from build123d import *
from build123d.topology import SkipClean

# Parameters (mm, degrees)
SKETCH1_R           = 7
BOSS_EXTRUDE1_DEPTH = 20
SKETCH2_R           = 13.25
CUT_EXTRUDE1_DEPTH  = 14
SKETCH3_R           = 4
CUT_EXTRUDE2_DEPTH  = 76.40989747
SKETCH4_W           = 110
SKETCH4_H           = 5
BOSS_EXTRUDE2_DEPTH = 10
SKETCH5_W           = 110
SKETCH5_H           = 5
BOSS_EXTRUDE3_DEPTH = 10
FILLET1_START       = -40
FILLET1_DEPTH       = 80
FILLET1_START_2     = -10.0000001
FILLET1_2_DEPTH     = 40.0000001
FILLET1_START_3     = -55.0000001
FILLET1_3_DEPTH     = 110.0000002
SKETCH6_R           = 2.5
CUT_EXTRUDE4_DEPTH  = 108.662433145
SKETCH8_R           = 40
CUT_EXTRUDE5_DEPTH  = 79.655277385


with BuildPart() as part:
    # Sketch1 → Boss-Extrude1 (new body)
    with BuildSketch(Plane(origin=(0, 0, 0), x_dir=(1, 0, 0), z_dir=(0, 1, 0))):
        with BuildLine():
            Line((-55, -42.556835854), (-40, -42.556835854))
            Line((-40, -42.556835854), (-40, 0))
            ThreePointArc((-40, 0), (0, 40), (40, 0))
            Line((40, 0), (40, -42.556835854))
            Line((40, -42.556835854), (55, -42.556835854))
            Line((55, -42.556835854), (55, -47.556835854))
            Line((55, -47.556835854), (-55, -47.556835854))
            Line((-55, -47.556835854), (-55, -42.556835854))
        make_face()
        with Locations(Location((0, 0, 0), (0, 0, 270))):
            Circle(SKETCH1_R, mode=Mode.SUBTRACT)
    extrude(amount=BOSS_EXTRUDE1_DEPTH)

    # Sketch2 → Cut-Extrude1 (cut)
    with BuildSketch(Plane(origin=(0, 20, 0), x_dir=(1, 0, 0), z_dir=(0, 1, 0))):
        with Locations(Location((0, 0, 0), (0, 0, 270))):
            Circle(SKETCH2_R)
    extrude(amount=-CUT_EXTRUDE1_DEPTH, mode=Mode.SUBTRACT)

    # Sketch3 → Cut-Extrude2 (cut, through all)
    with BuildSketch(Plane(origin=(0, 20, 0), x_dir=(1, 0, 0), z_dir=(0, 1, 0))):
        with Locations(Location((-21.213203436, 21.213203436, 0), (0, 0, 270))):
            Circle(SKETCH3_R)
        with Locations(Location((21.213203436, 21.213203436, 0), (0, 0, 270))):
            Circle(SKETCH3_R)
        with Locations(Location((21.213203436, -21.213203436, 0), (0, 0, 270))):
            Circle(SKETCH3_R)
        with Locations(Location((-21.213203436, -21.213203436, 0), (0, 0, 270))):
            Circle(SKETCH3_R)
    extrude(amount=-CUT_EXTRUDE2_DEPTH, mode=Mode.SUBTRACT)

    # Sketch4 → Boss-Extrude2 (add)
    with BuildSketch(Plane.XZ):
        with Locations((0, 45.056835854)):
            Rectangle(SKETCH4_W, SKETCH4_H)
    extrude(amount=BOSS_EXTRUDE2_DEPTH)

    # Sketch5 → Boss-Extrude3 (add)
    with BuildSketch(Plane(origin=(0, 20, 0), x_dir=(1, 0, 0), z_dir=(0, 1, 0))):
        with Locations((0, -45.056835854)):
            Rectangle(SKETCH5_W, SKETCH5_H)
    extrude(amount=BOSS_EXTRUDE3_DEPTH)

    # Fillet1: read off the stored shape, not the designer's step
    # Fillet1 outline → Fillet1 (add)
    with BuildSketch(Plane.YZ.offset(FILLET1_START)):
        with BuildLine():
            Line((0, 42.556835854), (-10, 42.556835854))
            add(Edge.make_bspline(
                [(-10, 42.556835854), (0, 42.556835854), (0, 32.556835854)],
                knots=[0, 0, 0, 1, 1, 1], degree=2, weights=[1, 0.707106781, 1]))
            Line((0, 32.556835854), (0, 42.556835854))
        make_face()
        with BuildLine():
            Line((30, 42.556835854), (20, 42.556835854))
            Line((20, 42.556835854), (20, 32.556835854))
            add(Edge.make_bspline(
                [(30, 42.556835854), (20, 42.556835854), (20, 32.556835854)],
                knots=[0, 0, 0, 1, 1, 1], degree=2, weights=[1, 0.707106781, 1]))
        make_face()
    extrude(amount=FILLET1_DEPTH)

    # Fillet1 2 outline → Fillet1 2 (add)
    with SkipClean():  # the faces are left unmerged after this step: merging them gives an invalid solid
        with BuildSketch(Plane(origin=(0, 0, 0), x_dir=(1, 0, 0), z_dir=(0, 1, 0)).offset(FILLET1_START_2)):
            with BuildLine():
                add(Edge.make_bspline(
                    [(40, -32.556835854), (40, -42.556835854), (50, -42.556835854)],
                    knots=[0, 0, 0, 1, 1, 1], degree=2, weights=[1, 0.707106781, 1]))
                Line((40, -32.556835854), (40, -42.556835854))
                Line((40, -42.556835854), (50, -42.556835854))
            make_face()
            with BuildLine():
                add(Edge.make_bspline(
                    [(-50, -42.556835854), (-40, -42.556835854), (-40, -32.556835854)],
                    knots=[0, 0, 0, 1, 1, 1], degree=2, weights=[1, 0.707106781, 1]))
                Line((-50, -42.556835854), (-40, -42.556835854))
                Line((-40, -42.556835854), (-40, -32.556835854))
            make_face()
        extrude(amount=FILLET1_2_DEPTH)

    # Fillet1 3 outline → Fillet1 3 (cut)
    with BuildSketch(Plane.YZ.offset(FILLET1_START_3)):
        with BuildLine():
            Line((-10, 42.556835854), (-10.0000001, 32.556835854))
            Line((-10.0000001, 32.556835854), (0, 32.556835854))
            add(Edge.make_bspline(
                [(-10, 42.556835854), (0, 42.556835854), (0, 32.556835854)],
                knots=[0, 0, 0, 1, 1, 1], degree=2, weights=[1, 0.707106781, 1]))
        make_face()
        with BuildLine():
            add(Edge.make_bspline(
                [(30, 42.556835854), (20, 42.556835854), (20, 32.556835854)],
                knots=[0, 0, 0, 1, 1, 1], degree=2, weights=[1, 0.707106781, 1]))
            Line((20, 32.556835854), (30, 32.556835854))
            Line((30, 32.556835854), (30, 42.556835854))
        make_face()
    extrude(amount=FILLET1_3_DEPTH, mode=Mode.SUBTRACT)

    # Sketch6 → Cut-Extrude4 (cut, through all)
    with BuildSketch(Plane.XY.offset(47.556835854)):
        with Locations((-47.5, 20)):
            Circle(SKETCH6_R)
        with Locations(Location((-47.5, 0, 0), (0, 0, 180))):
            Circle(SKETCH6_R)
        with Locations((47.5, 0)):
            Circle(SKETCH6_R)
        with Locations((47.5, 20)):
            Circle(SKETCH6_R)
    extrude(amount=-CUT_EXTRUDE4_DEPTH, mode=Mode.SUBTRACT)

    # Sketch8 → Cut-Extrude5 (cut, through all)
    with BuildSketch(Plane(origin=(0, 20, 0), x_dir=(1, 0, 0), z_dir=(0, 1, 0))):
        Circle(SKETCH8_R)
    extrude(amount=CUT_EXTRUDE5_DEPTH, mode=Mode.SUBTRACT)


solid = part.part
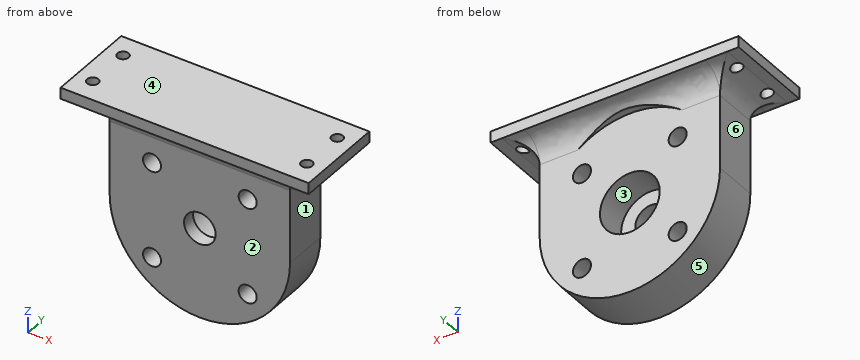
Here's how the part is built. I have some questions about the finished solid (model axes, mm). Face numbers are marked on the shaded views. A direction names the side the tool comes from. Round coordinates to 2 decimals unless told otherwise and drop trailing zeros. Order: outer loops, then holes, each group sorted by start corner. A loop starts at its lowest first (then second) coordinate and runs counter-clockwise, first axis right, second up. Notation, with made-up numbers: (-19, 63) -> (-2, 63) arc R16 cw to (-2, 93) -> close; hole circle Ø4 at (16, 46). An arc over 180 degrees is marked (long way). Use CSV: the item, a comma, the result in double quotes.
1. I want a section at B-B on x = -47.5. Give the number of separate pieces and of enclosed holes in the cut face, and give its area (3 significant figures).
Recorded:
separate pieces,"3"
enclosed holes,"0"
area,"158 mm2"
2. I need wall thicknesses on line 1 along X through (y, z) = (20, 43); line 2 along X through (y, z) = (0.5, 19); line 3 along Y through (x, z) = (-47, 44). Which ranges of each line are inside material? Lowest first, please.
Recorded:
line 1,"x = -55 to -50, -45 to 45, 50 to 55"
line 2,"x = -40 to -24.55, -17.88 to 17.88, 24.55 to 40"
line 3,"y = -10 to -2.45, 2.45 to 17.55, 22.45 to 30"
3. Which directions (+Z, -Z, +X, -X, +Y, -Y) give clear straight access to the entire face, cutting with the end or side of a thin tool? Please do the marked faces 1 and 2.
Recorded:
face 1,"-Z, +X, +Y, -Y"
face 2,"-Z, +X, -X, -Y"
4. I want a section at D-D on z = -32.5. List the corners of the cut face in (x, y) for me, and give its area (3 significant figures).
Recorded:
outline,"(-23.32, 0) -> (23.32, 0) -> (23.32, 20) -> (-23.32, 20) -> close"
area,"933 mm2"
5. I'm going to push flat-ended pins straight in: P1, Ø4, axis at x = -47.5, y = 20, coming from the +Z side; P2, Ø10.5, axis at x = 21.21, z = 21.21, coming from the +Y side; P3, Ø12, axis at y = 18.5, z = -1, coming from the -X side; P4, Ø8, axis at x = 47.5, y = 0, coming from the -Z side. Where does each tip first touch, or does it pass through?
Recorded:
P1,"passes through"
P2,"stops at y = 20"
P3,"stops at x = -40"
P4,"stops at z = 40.16"
6. I want a section at A-A on z = -3.5. List the corners of the cut face in (x, y) for me, and give its area (3 significant figures).
Recorded:
outline,"(-39.85, 0) -> (-6.06, 0) -> (-6.06, 6) -> (-12.78, 6) -> (-12.78, 20) -> (-39.85, 20) -> close; (6.06, 0) -> (39.85, 0) -> (39.85, 20) -> (12.78, 20) -> (12.78, 6) -> (6.06, 6) -> close"
area,"1,160 mm2"
7. Thinking about a two-plate mould opening in Z: for the marked faces 3, 4, 5 and 6, which applies, pulls with the +Z half, pulls with the -Z half, needs draft (parallel to the pull), parting line crosses it, or undercut?
Recorded:
face 3,"undercut"
face 4,"pulls with the +Z half"
face 5,"pulls with the -Z half"
face 6,"needs draft"
